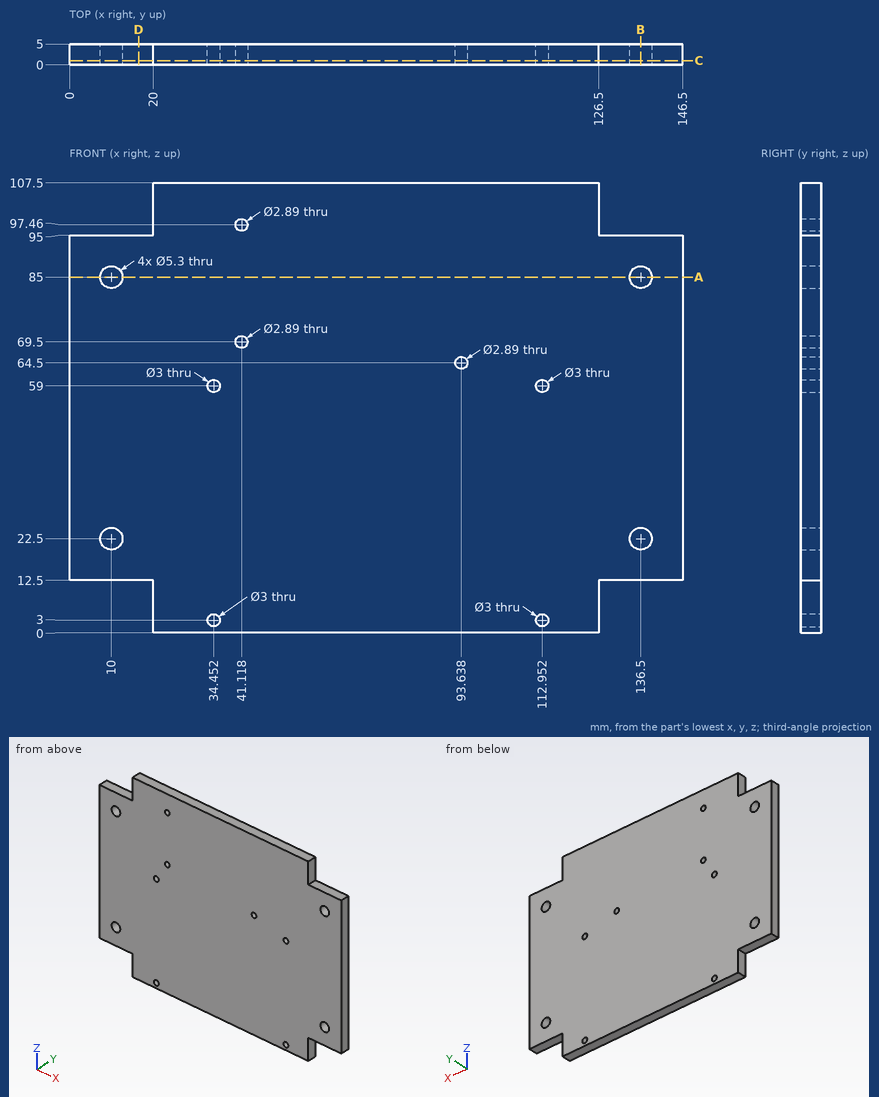
Here's the drawing with two shaded views (mm, measured from the low corner). I have some questions. Coordinates: 2 decimals unless noted, no trailing zeros. Write each loop counter-clockwise with the first axis right and the second up, starting at its lowest first coordinate (ties: lowest second). Pieces come first, ordered by that corner, then holes. Notation, with made-up numbers: (22, 43) -> (36, 43) arc R14 cw to (36, 66) -> close; hole circle Ø11 at (46.5, 17). An arc over 180 degrees is marked (long way). Use a Markdown table: item, result. Add a question column.
(1) If we section it at D-D, the plane x = 16.5: Write out the boundary of the cut face in (y, z).
(2) If we section it at A-A, the plane z = 85: Write out the boundary of the cut face in (x, y).
(3) If we section it at B-B, the plane x = 136.5: Write out the boundary of the cut face in (y, z).
(4) I'm going to push flat-ended pins straight in: P1, Ø2.5, axis at y = 3.5, z = 102.5, coming from the +X side; P2, Ø2.5, axis at x = 138.5, y = 1.5, coming from the -Z side; P3, Ø2.5, axis at x = 5.5, y = 2.5, coming from the +Z side. Where does each tip first touch, or does it pass through?
(5) Please list where these lines run through material, in increasing order: line 1 (X direction, y = 3.05, z = 22.5); line 2 (X direction, y = 1.5, z = 3); line 3 (Z direction, x = 136.5, y = 2.15).
(6) If we section it at C-C, the plane y = 1: State how many separate pieces and enclosed holes the cut face has, and give its area (3 significant figures).
Outcome:
| question | item | result |
|---|---|---|
| 1 | outline | (0, 12.5) -> (5, 12.5) -> (5, 95) -> (0, 95) -> close |
| 2 | outline | (0, 0) -> (7.35, 0) -> (7.35, 5) -> (0, 5) -> close; (12.65, 0) -> (133.85, 0) -> (133.85, 5) -> (12.65, 5) -> close; (139.15, 0) -> (146.5, 0) -> (146.5, 5) -> (139.15, 5) -> close |
| 3 | outline | (0, 12.5) -> (5, 12.5) -> (5, 19.85) -> (0, 19.85) -> close; (0, 25.15) -> (5, 25.15) -> (5, 82.35) -> (0, 82.35) -> close; (0, 87.65) -> (5, 87.65) -> (5, 95) -> (0, 95) -> close |
| 4 | P1 | stops at x = 126.5 |
| 4 | P2 | stops at z = 12.5 |
| 4 | P3 | stops at z = 95 |
| 5 | line 1 | x = 0 to 7.35, 12.65 to 133.85, 139.15 to 146.5 |
| 5 | line 2 | x = 20 to 32.95, 35.95 to 111.45, 114.45 to 126.5 |
| 5 | line 3 | z = 12.5 to 19.85, 25.15 to 82.35, 87.65 to 95 |
| 6 | separate pieces | 1 |
| 6 | enclosed holes | 11 |
| 6 | area | 14,600 mm^2 |
